from build123d import *

# Parameters (mm, degrees)
F0_R     = 6
F0_R_2   = 2
F1_DEPTH = 20
F2_T     = -1
F3_DEPTH = 25
F4_R     = 1
F5_R     = 0.49999


# Not quite as in the source:
# - a fillet or chamfer is up to 0.001 mm smaller than in the source, because OpenCascade refuses the exact size


with BuildPart() as f1:
    # F0 (on Top) → F1 (new body)
    with BuildSketch(Plane.XY):
        Circle(F0_R)
        Circle(F0_R_2, mode=Mode.SUBTRACT)
        Circle(F0_R_2)
    extrude(amount=F1_DEPTH)

    # F2
    f2_openings = [f1.faces().sort_by_distance(p)[0] for p in [
        (0, 0, 20),
    ]]
    offset(amount=F2_T, openings=f2_openings)

    # F0 (on Top) → F3 (cut)
    with BuildSketch(Plane.XY):
        Circle(F0_R_2)
    extrude(amount=F3_DEPTH, mode=Mode.SUBTRACT)

    # F4
    f4_edges = [f1.edges().sort_by_distance(p)[0] for p in [
        (-6, 0, 0),
        (-5, 0, 1),
    ]]
    fillet(f4_edges, radius=F4_R)

    # F5 (radius 0.5 in the source; OpenCascade refuses exactly that, so slightly less here)
    f5_edges = [f1.edges().sort_by_distance(p)[0] for p in [
        (-5, 0, 20),
        (-6, 0, 20),
    ]]
    fillet(f5_edges, radius=F5_R)


solid = f1.part
Check sheet for the modelled part. Datum: model origin and axes. Units: mm. A direction names the side the tool comes from. Round coordinates to 2 decimals unless told otherwise and drop trailing zeros. Loops run counter-clockwise (first coordinate to the right, second up) from the corner with the lowest first, then second, coordinate; pieces in that order, holes last. Notation, with made-up numbers: (-6, -6.5) - (51, -6.5) arc R27 ccw to (51, 16.5) - close; hole circle Ø11 at (55, 33). An arc over 180 degrees is marked (long way). Answer as CSV lines item,"result". Start each with the question number.
Item 1: Section check C-C (z = 15.5). Record the boundary of the cut face in (x, y), and give its area (3 significant figures).
Item 2: Release check for a two-part mould opening along X. For faces 1 (the cylindrical face through (-1.08, -4.88, 10.63)), 2 (the flat face through (-0.1, -2.2, 0)), 3 (the cylindrical face through (-6, 0, 10)) record: +X half, -X half, draft (parallel to the pull), parting line (faces both ways), or undercut.
Item 3: Depth check by flat-ended pin: P1, Ø2.5, axis at x = 2, y = -2, coming from the +Z side; P2, Ø2.5, axis at x = 0, y = 0, coming from the +Z side; P3, Ø1, axis at y = 3.5, z = 6, coming from the -X side. Enter the tip coordinate at first touch or a pass-through.
Item 4: Set-up check for faces 4 (the cylindrical face through (-0.434, -1.952, 0.493)), 5 (the flat face through (-2, -1, 1)): record each of +Z, -Z, +X, -X, +Y, -Y from which the full face is reachable in a straight line by a thin tool's end or side.
Item 5: Scan lines: line 1 (Z direction, x = 0, y = -2.5); line 2 (Y direction, x = 0, z = 14.75); line 3 (Y direction, x = -1.5, z = 19). Record each from-to range of solid material in increasing order. Write a range as [from, to].
Report:
1,outline,"circle Ø12 at (0, 0); hole circle Ø10 at (0, 0)"
1,area,"34.6 mm2"
2,face 1,"undercut"
2,face 2,"draft"
2,face 3,"parting line"
3,P1,"stops at z = 1"
3,P2,"passes through"
3,P3,"stops at x = -5.2"
4,face 4,"+Z, -Z"
4,face 5,"+Z"
5,line 1,"z = [0, 1]"
5,line 2,"y = [-6, -5], [5, 6]"
5,line 3,"y = [-5.81, -4.77], [4.77, 5.81]"
